Could you check a few things on this model? Use its own coordinates, in mm. A direction names the side the tool comes from. Coordinates: 2 decimals unless noted, no trailing zeros. Write each loop counter-clockwise with the first axis right and the second up, starting at its lowest first coordinate (ties: lowest second). Pieces come first, ordered by that corner, then holes.
Item 1: I want a section at C-C on y = 15. Please give me the cut outline in (x, z), then the cut area to 3 significant figures.
Item 2: I want a section at A-A on y = 23. Please give me the cut outline in (x, z).
Item 3: I want a section at B-B on z = 2.8. Please give me the cut outline in (x, y) (3 decimals), then the cut area to 3 significant figures.
Item 4: For P1, Ø1.2, axis at y = 32, z = 1.5, coming from the +X side; P2, Ø1.8, axis at x = 11, y = 5.15, coming from the -Z side; P3, Ø2.5, axis at x = 129, y = 29.85, coming from the +Z side; P4, Ø1.2, axis at y = 32, z = 1, coming from the -X side, each with a flat end and sliding along its axis, tell me the tip position at first contact or that it passes through.
Item 5: Thinking about a two-plate mould opening in X: for faces 5 (the cylindrical face through (-12.347, 17.772, 1.972)), 6 (the flat face through (19, 29.85, 2)), 7 (the flat face through (69, 18, 0)), which applies, +X half, -X half, draft (parallel to the pull), parting line (faces both ways), or undercut?
Item 6: If I drill on probe 1 along Y at (x, z) = (129, 0.95); probe 2 along X at (y, z) = (30, 0.6); probe 3 along X at (y, z) = (4.5, 3.85), over which ranges is the centre line in solid material (lowest first)?
Item 7: Which directions (+Z, -Z, +X, -X, +Y, -Y) give clear straight access to the entire face, cutting with the end or side of a thin tool? Please do faces 1 (the flat face through (0, 3, 2)), 2 (the flat face through (140, 32, 2)), 3 (the flat face through (0, 32, 2)), 4 (the flat face through (24, 17, 2)).
from build123d import *

# Parameters (mm, degrees)
SKETCH_R    = 1
SKETCH_W    = 10
SKETCH_H    = 24.7
PAD_DEPTH   = 4
FILLET_R    = 1
FILLET001_R = 1
FILLET002_R = 1
FILLET003_R = 1
FILLET004_R = 2
FILLET005_R = 2
FILLET006_R = 2
FILLET007_R = 2


with BuildPart() as part:
    # Sketch → Pad (new body)
    with BuildSketch(Plane.XY):
        with BuildLine():
            Line((0, 0), (140, 0))
            Line((140, 5.15), (140, 0))
            ThreePointArc((140, 5.15), (152.35, 17.5), (140, 29.85))
            Line((140, 35), (140, 29.85))
            Line((140, 35), (0, 35))
            Line((0, 35), (0, 29.85))
            ThreePointArc((0, 29.85), (-12.35, 17.5), (0, 5.15))
            Line((0, 5.15), (0, 0))
        make_face()
        with Locations((129, 29.85)):
            Circle(SKETCH_R, mode=Mode.SUBTRACT)
        with Locations((129, 5.15)):
            Circle(SKETCH_R, mode=Mode.SUBTRACT)
        with Locations((11, 29.85)):
            Circle(SKETCH_R, mode=Mode.SUBTRACT)
        with Locations((11, 5.15)):
            Circle(SKETCH_R, mode=Mode.SUBTRACT)
        with Locations((-6.175, 17.5)):
            Circle(SKETCH_R, mode=Mode.SUBTRACT)
        with Locations((146.175, 17.5)):
            Circle(SKETCH_R, mode=Mode.SUBTRACT)
        with Locations((19, 17.5)):
            Rectangle(SKETCH_W, SKETCH_H, mode=Mode.SUBTRACT)
    extrude(amount=PAD_DEPTH)

    # Fillet
    fillet_edges = [part.edges().sort_by_distance(p)[0] for p in [
        (140, 0, 2),
    ]]
    fillet(fillet_edges, radius=FILLET_R)

    # Fillet001
    fillet001_edges = [part.edges().sort_by_distance(p)[0] for p in [
        (0, 0, 2),
    ]]
    fillet(fillet001_edges, radius=FILLET001_R)

    # Fillet002
    fillet002_edges = [part.edges().sort_by_distance(p)[0] for p in [
        (140, 35, 2),
    ]]
    fillet(fillet002_edges, radius=FILLET002_R)

    # Fillet003
    fillet003_edges = [part.edges().sort_by_distance(p)[0] for p in [
        (0, 35, 2),
    ]]
    fillet(fillet003_edges, radius=FILLET003_R)

    # Fillet004
    fillet004_edges = [part.edges().sort_by_distance(p)[0] for p in [
        (14, 29.85, 2),
    ]]
    fillet(fillet004_edges, radius=FILLET004_R)

    # Fillet005
    fillet005_edges = [part.edges().sort_by_distance(p)[0] for p in [
        (14, 5.15, 2),
    ]]
    fillet(fillet005_edges, radius=FILLET005_R)

    # Fillet006
    fillet006_edges = [part.edges().sort_by_distance(p)[0] for p in [
        (24, 5.15, 2),
    ]]
    fillet(fillet006_edges, radius=FILLET006_R)

    # Fillet007
    fillet007_edges = [part.edges().sort_by_distance(p)[0] for p in [
        (24, 29.85, 2),
    ]]
    fillet(fillet007_edges, radius=FILLET007_R)


solid = part.part
Response values:
1. outline: (-12.09, 0) - (14, 0) - (14, 4) - (-12.09, 4) - close; (24, 0) - (152.09, 0) - (152.09, 4) - (24, 4) - close
1. area: 617 mm2
2. outline: (-11.06, 0) - (14, 0) - (14, 4) - (-11.06, 4) - close; (24, 0) - (151.06, 0) - (151.06, 4) - (24, 4) - close
3. outline: (0, 1) arc R1 ccw to (1, 0) - (139, 0) arc R1 ccw to (140, 1) - (140, 5.15) arc R12.35 ccw to (140, 29.85) - (140, 34) arc R1 ccw to (139, 35) - (1, 35) arc R1 ccw to (0, 34) - (0, 29.85) arc R12.35 ccw to (0, 5.15) - close; hole circle Ø2 at (-6.175, 17.5); hole circle Ø2 at (11, 5.15); hole circle Ø2 at (11, 29.85); hole (14, 7.15) arc R2 ccw to (16, 5.15) - (22, 5.15) arc R2 ccw to (24, 7.15) - (24, 27.85) arc R2 ccw to (22, 29.85) - (16, 29.85) arc R2 ccw to (14, 27.85) - close; hole circle Ø2 at (129, 5.15); hole circle Ø2 at (129, 29.85); hole circle Ø2 at (146.175, 17.5)
3. area: 5,120 mm2
4. P1: stops at x = 140
4. P2: passes through
4. P3: stops at z = 4
4. P4: stops at x = 0
5. face 5: -X half
5. face 6: undercut
5. face 7: draft
6. probe 1: y = 0 to 4.15, 6.15 to 28.85, 30.85 to 35
6. probe 2: x = 0 to 10.01, 11.99 to 128.01, 129.99 to 140
6. probe 3: x = 0 to 10.24, 11.76 to 128.24, 129.76 to 140
7. face 1: +Z, -Z, -X, -Y
7. face 2: +Z, -Z, +X, +Y
7. face 3: +Z, -Z, -X, +Y
7. face 4: +Z, -Z
